```python
from build123d import *

# Parameters (mm, degrees)
F0_R      = 60
F0_R_2    = 40
F3_DEPTH  = 3
F4_R      = 60
F4_R_2    = 40
F5_DEPTH  = 2
F9_R      = 3
F10_R     = 0.75
F11_DEPTH = 50.001


# Not quite as in the source:
# - a fillet or chamfer that OpenCascade refuses, or shapes differently, is made with other operations: its cross-section is extruded or revolved along the edge and cut away or added


with BuildPart() as f3:
    # F0 (on Top) → F3 (new body)
    with BuildSketch(Plane.XY):
        Circle(F0_R)
        Polygon((-25, -34.4095480118), (-25, -42.9095480118), (-31.175611488, -42.9095480118), (-33.0839803885, -37.036192464), align=None, mode=Mode.SUBTRACT)
        Polygon((25, -34.4095480118), (33.0839803885, -37.036192464), (31.175611488, -42.9095480118), (25, -42.9095480118), align=None, mode=Mode.SUBTRACT)
        Polygon((-45.4470243632, 20.0199222552), (-40.4508497187, 13.143277803), (-48.5348301073, 10.5166333508), (-50.4431990077, 16.3899888986), align=None, mode=Mode.SUBTRACT)
        Circle(F0_R_2, mode=Mode.SUBTRACT)
        Polygon((50.4431990077, 16.3899888986), (48.5348301073, 10.5166333508), (40.4508497187, 13.143277803), (45.4470243632, 20.0199222552), align=None, mode=Mode.SUBTRACT)
        Polygon((4.9961746445, 49.4091848698), (0, 42.5325404176), (-4.9961746445, 49.4091848698), (0, 53.0391182264), align=None, mode=Mode.SUBTRACT)
    extrude(amount=F3_DEPTH)

    # F4 (on face) → F5 (join)
    with BuildSketch(Plane.XY.offset(3)):
        Circle(F4_R)
        Polygon((-31.175611488, -42.9095480118), (-33.0839803885, -37.036192464), (-25, -34.4095480118), (-25, -42.9095480118), align=None, mode=Mode.SUBTRACT)
        Polygon((25, -42.9095480118), (25, -34.4095480118), (33.0839803885, -37.036192464), (31.175611488, -42.9095480118), align=None, mode=Mode.SUBTRACT)
        Polygon((-40.4508497187, 13.143277803), (-48.5348301073, 10.5166333508), (-50.4431990077, 16.3899888986), (-45.4470243632, 20.0199222552), align=None, mode=Mode.SUBTRACT)
        Circle(F4_R_2, mode=Mode.SUBTRACT)
        Polygon((40.4508497187, 13.143277803), (45.4470243632, 20.0199222552), (50.4431990077, 16.3899888986), (48.5348301073, 10.5166333508), align=None, mode=Mode.SUBTRACT)
        Polygon((0, 53.0391182264), (4.9961746445, 49.4091848698), (0, 42.5325404176), (-4.9961746445, 49.4091848698), align=None, mode=Mode.SUBTRACT)
        Polygon((-50.4431990077, 16.3899888986), (-48.5348301073, 10.5166333508), (-40.4508497187, 13.143277803), (-45.4470243632, 20.0199222552), align=None)
        Polygon((0, 42.5325404176), (4.9961746445, 49.4091848698), (0, 53.0391182264), (-4.9961746445, 49.4091848698), align=None)
        Polygon((50.4431990077, 16.3899888986), (45.4470243632, 20.0199222552), (40.4508497187, 13.143277803), (48.5348301073, 10.5166333508), align=None)
        Polygon((33.0839803885, -37.036192464), (25, -34.4095480118), (25, -42.9095480118), (31.175611488, -42.9095480118), align=None)
        Polygon((-25, -34.4095480118), (-33.0839803885, -37.036192464), (-31.175611488, -42.9095480118), (-25, -42.9095480118), align=None)
    extrude(amount=F5_DEPTH)

    # F6 (on Front) → F8 (revolve)
    with BuildSketch(Plane.XZ):
        Polygon((-1.5, 50), (-60, 5), (-40.3058288648, 5), (0, 47), (0, 50), align=None)
    revolve(axis=Axis((0, 0, 19.0761145204), (0, 0, 1)))

    # F9
    f9_edges = [f3.edges().sort_by_distance(p)[0] for p in [
        (0, -60, 5),
        (0, 60, 5),
        (-60, 0, 0),
    ]]
    fillet(f9_edges, radius=F9_R)

    # F10 (on offset) → F11 (cut, through all)
    with BuildSketch(Plane.XY.offset(50)):
        Circle(F10_R)
    extrude(amount=-F11_DEPTH, mode=Mode.SUBTRACT)

    # F12: fillet of radius 5 on 1 edges, made by hand

    # F12_s1 → F12_t2 (revolve, cut)
    with BuildSketch(Plane.XZ):
        with BuildLine():
            ThreePointArc((40, 3.2781529238), (40.0770509003, 4.1525510952), (40.3058288648, 5))
            Line((40.3058288648, 5), (40.2119454421, 5.0344369415))
            ThreePointArc((40.2119454421, 5.0344369415), (40.1529144324, 5.1), (40, 5.1))
            Line((40, 5.1), (39.9, 5))
            Line((39.9, 5), (39.9, 3.2781529238))
            Line((39.9, 3.2781529238), (40, 3.2781529238))
        make_face()
    revolve(axis=Axis((0, 0, 5), (0, 0, 1)), mode=Mode.SUBTRACT)


solid = f3.part
```
The listing builds one solid part. Answer for the finished solid, in the listing's coordinates (mm). A direction names the side the tool comes from. Give positions to 0.01 mm unless a question says otherwise; leave off trailing zeros. Order: outer loops, then holes, each group sorted by start corner. A loop starts at its lowest first (then second) coordinate and runs counter-clockwise, first axis right, second up.
1) For faces 4 (the face through (-10.93, -3.44, 42.34)), 5 (the face through (-29.1, -35.74, 1.48)), determine the directions among +Z, -Z, +X, -X, +Y, -Y from which every point of the face is accessible in a straight line to the end or side of a thin tool.
Reported:
face 4: +Z
face 5: -Z
2) Find section A-A on z = 44. Write down the section's boundary in (x, y).
Reported:
outline: circle Ø18.6 at (0, 0); hole circle Ø5.76 at (0, 0)
3) Determine the mould class of faces 1 (the face through (12, 39, 0)), 2 (the face through (-59.94, 2.64, 3.26)), 3 (the face through (-25, -39, 1)) for opening direction Y: pulls with the +Y half, pulls with the -Y half, needs draft (parallel to the pull), parting line crosses it, or undercut.
Reported:
face 1: needs draft
face 2: parting line crosses it
face 3: undercut
4) Consider line 1 along Y through (x, z) = (0, 48.4); line 2 along Y through (x, z) = (0, 47); line 3 along X through (y, z) = (31, 7). Determine where each line is inside the solid, lowest interval first.
Reported:
line 1: y = -3.58 to -0.75, 0.75 to 3.58
line 2: y = -5.4 to -0.75, 0.75 to 5.4
line 3: x = -48.31 to -22.64, 22.64 to 48.31
5) Find section B-B on z = 11.5. Write down the section's boundary in (x, y).
Reported:
outline: circle Ø103.1 at (0, 0); hole circle Ø68.14 at (0, 0)
6) Given P1, Ø9, axis at x = 30.5, y = -38, coming from the -Z side; P2, Ø3.5, axis at x = 29, z = 2, coming from the +Y side; P3, Ø3, axis at x = -42, y = 12.5, coming from the +Z side; P4, Ø1.5, axis at y = -39.5, z = 1.5, coming from the -X side, each flat-ended and moving along its own axis, determine where each tip first touches the part or whether it passes through.
Reported:
P1: stops at z = 0
P2: stops at y = 53.37
P3: stops at z = 18.6
P4: stops at x = -45.44
